For this review, take the finished solid that the model builds, in its own axes (mm). Face numbers are marked on the shaded views. Coordinates: 2 decimals unless noted, no trailing zeros. Write each loop counter-clockwise with the first axis right and the second up, starting at its lowest first coordinate (ties: lowest second). Pieces come first, ordered by that corner, then holes. Notation, with made-up numbers: (-2, 37.25) - (25, 37.25) arc R17 cw to (25, 64.25) - close; hole circle Ø2 at (-28, 1.25). An arc over 180 degrees is marked (long way). Use one line per item in the form item = value. Start each with the question number.
1) We need section A-A (z = 0). Give the boundary of the cut face in (x, y) (3 decimals), plus the area to 4 significant figures.
2) Mouldability with a two-part tool opening along Z and no side actions: class the marked faces 1 and 2 as pulls with the +Z half, pulls with the -Z half, needs draft (parallel to the pull), parting line crosses it, or undercut.
3) Insertion check: P1, Ø12, axis at x = -21, y = 22.5, coming from the +Z side; P2, Ø0.8, axis at x = -33.5, z = 4.5, coming from the -Y side; P3, Ø8, axis at x = 17, y = 23, coming from the +Z side; P4, Ø0.8, axis at x = -33, y = 15, coming from the +Z side. Each pin has a flat end and moves straight along its axis. Give the tip position at first contact, or say it passes through.
4) We need section C-C (y = 10). Give the boundary of the cut face in (x, z) (3 decimals), plus the area to 3 significant figures.
5) We need section B-B (x = 8). Give the boundary of the cut face in (y, z).
6) For L1, parallel to Z at x = 0, y = 23 (3 decimals); L2, parallel to X at y = 19, z = 0 (3 decimals), list the stretches that pass through material, from the lowest coordinate up. Write a range as from..to.
```python
from build123d import *

# Parameters (mm, degrees)
SKETCH1_R           = 35.375
SKETCH1_R_2         = 34.375
BOSS_EXTRUDE1_DEPTH = 31.75
SKETCH2_W           = 22
SKETCH2_H           = 24.25
CUT_EXTRUDE1_DEPTH  = 43


with BuildPart() as part:
    # Sketch1 → Boss-Extrude1 (new body)
    with BuildSketch(Plane(origin=(0, 0, 0), x_dir=(1, 0, 0), z_dir=(0, 1, 0))):
        Circle(SKETCH1_R)
        Circle(SKETCH1_R_2, mode=Mode.SUBTRACT)
    extrude(amount=BOSS_EXTRUDE1_DEPTH)

    # Sketch2 → Cut-Extrude1 (cut)
    with BuildSketch(Plane(origin=(0, 0, 0), x_dir=(0, 0, -1), z_dir=(1, 0, 0))):
        with Locations((0, 12.125)):
            Rectangle(SKETCH2_W, SKETCH2_H)
    extrude(amount=-CUT_EXTRUDE1_DEPTH, mode=Mode.SUBTRACT)


solid = part.part
```
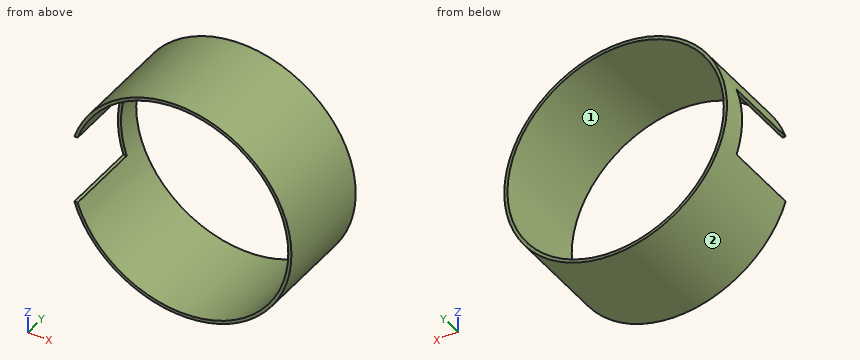
Determined:
q1.outline = (-35.375, 24.25) - (-34.375, 24.25) - (-34.375, 31.75) - (-35.375, 31.75) - close; (34.375, 0) - (35.375, 0) - (35.375, 31.75) - (34.375, 31.75) - close
q1.area = 39.25 mm²
q2.face_1 = undercut
q2.face_2 = parting line crosses it
q3.P1 = 32.04
q3.P2 = through
q3.P3 = 32.9
q3.P4 = 13.73
q4.outline = (-33.621, -11) arc R35.375 ccw (long way) to (-33.621, 11) - (-32.567, 11) arc R34.375 cw (long way) to (-32.567, -11) - close
q4.area = 197 mm²
q5.outline = (0, -34.46) - (31.75, -34.46) - (31.75, -33.43) - (0, -33.43) - close; (0, 33.43) - (31.75, 33.43) - (31.75, 34.46) - (0, 34.46) - close
q6.L1 = -35.375..-34.375, 34.375..35.375
q6.L2 = 34.375..35.375
